Source: CAD feature listing. Evaluate the final solid. Frame: model axes, mm. A direction names the side the tool comes from. Coordinates: 2 decimals unless noted, no trailing zeros. Write each loop counter-clockwise with the first axis right and the second up, starting at its lowest first coordinate (ties: lowest second). Pieces come first, ordered by that corner, then holes. Notation, with made-up numbers: (76, -19) - (118, -19) arc R30 cw to (118, 13) - close; hole circle Ø1 at (0.25, 78). An arc over 180 degrees is marked (long way). One line per item, written item: value.
from build123d import *

# Parameters (mm, degrees)
F1_DEPTH  = 5.5372
F3_D      = 57.8866
F5_DEPTH  = 5.5382
F7_DEPTH  = 17.76331
F9_DEPTH  = 25.4
F11_DEPTH = 25.4
F13_DEPTH = 25.4


with BuildPart() as f1:
    # F0 (on Front) → F1 (new body)
    with BuildSketch(Plane.XZ):
        Polygon((85.176131, 104.177512), (-67.223869, 104.177512), (-143.423869, -1.364378), (-143.423869, -52.164378), (161.376131, -52.164378), (161.376131, -1.364378), align=None)
    extrude(amount=F1_DEPTH)

    # F3 (through all)
    with Locations(Plane.XZ.offset(5.5372)):
        with Locations((-41.244327, 53.377512), (59.196589, 53.377512), (110.576131, 2.577512), (8.976131, 2.577512), (-92.623869, 2.577512)):
            Hole(F3_D / 2)

    # F4 (on face) → F5 (cut, through all)
    with BuildSketch(Plane.XZ.offset(5.5372)):
        with BuildLine():
            ThreePointArc((-87.315269, -35.095578), (-88.140769, -34.270078), (-88.966269, -35.095578))
            Line((-88.966269, -35.095578), (-88.966269, -43.985578))
            Line((-88.966269, -43.985578), (-71.516469, -43.985578))
            Line((-71.516469, -43.985578), (-71.516469, -35.095578))
            ThreePointArc((-71.516469, -35.095578), (-72.341969, -34.270078), (-73.167469, -35.095578))
            Line((-73.167469, -35.095578), (-73.167469, -41.597978))
            Line((-73.167469, -41.597978), (-87.315269, -41.597978))
            Line((-87.315269, -41.597978), (-87.315269, -35.095578))
        make_face()
    extrude(amount=-F5_DEPTH, mode=Mode.SUBTRACT)

    # F6 (on face) → F7 (cut)
    with BuildSketch(Plane.XZ.offset(5.5372)):
        with BuildLine():
            ThreePointArc((-43.424069, -35.095578), (-44.249569, -34.270078), (-45.075069, -35.095578))
            Line((-45.075069, -35.095578), (-45.075069, -43.985578))
            Line((-45.075069, -43.985578), (-27.625269, -43.985578))
            Line((-27.625269, -43.985578), (-27.625269, -35.095578))
            ThreePointArc((-27.625269, -35.095578), (-28.450769, -34.270078), (-29.276269, -35.095578))
            Line((-29.276269, -35.095578), (-29.276269, -41.597978))
            Line((-29.276269, -41.597978), (-43.424069, -41.597978))
            Line((-43.424069, -41.597978), (-43.424069, -35.095578))
        make_face()
    extrude(amount=-F7_DEPTH, mode=Mode.SUBTRACT)

    # F8 (on face) → F9 (cut)
    with BuildSketch(Plane.XZ.offset(5.5372)):
        with BuildLine():
            ThreePointArc((1.076731, -35.095578), (0.251231, -34.270078), (-0.574269, -35.095578))
            Line((-0.574269, -35.095578), (-0.574269, -43.985578))
            Line((-0.574269, -43.985578), (16.875531, -43.985578))
            Line((16.875531, -43.985578), (16.875531, -35.095578))
            ThreePointArc((16.875531, -35.095578), (16.050031, -34.270078), (15.224531, -35.095578))
            Line((15.224531, -35.095578), (15.224531, -41.597978))
            Line((15.224531, -41.597978), (1.076731, -41.597978))
            Line((1.076731, -41.597978), (1.076731, -35.095578))
        make_face()
    extrude(amount=-F9_DEPTH, mode=Mode.SUBTRACT)

    # F10 (on face) → F11 (cut)
    with BuildSketch(Plane.XZ.offset(5.5372)):
        with BuildLine():
            ThreePointArc((47.228531, -35.095578), (46.403031, -34.270078), (45.577531, -35.095578))
            Line((45.577531, -35.095578), (45.577531, -43.985578))
            Line((45.577531, -43.985578), (63.027331, -43.985578))
            Line((63.027331, -43.985578), (63.027331, -35.095578))
            ThreePointArc((63.027331, -35.095578), (62.201831, -34.270078), (61.376331, -35.095578))
            Line((61.376331, -35.095578), (61.376331, -41.597978))
            Line((61.376331, -41.597978), (47.228531, -41.597978))
            Line((47.228531, -41.597978), (47.228531, -35.095578))
        make_face()
    extrude(amount=-F11_DEPTH, mode=Mode.SUBTRACT)

    # F12 (on face) → F13 (cut)
    with BuildSketch(Plane.XZ.offset(5.5372)):
        with BuildLine():
            ThreePointArc((91.119731, -35.095578), (90.294231, -34.270078), (89.468731, -35.095578))
            Line((89.468731, -35.095578), (89.468731, -43.985578))
            Line((89.468731, -43.985578), (106.918531, -43.985578))
            Line((106.918531, -43.985578), (106.918531, -35.095578))
            ThreePointArc((106.918531, -35.095578), (106.093031, -34.270078), (105.267531, -35.095578))
            Line((105.267531, -35.095578), (105.267531, -41.597978))
            Line((105.267531, -41.597978), (91.119731, -41.597978))
            Line((91.119731, -41.597978), (91.119731, -35.095578))
        make_face()
    extrude(amount=-F13_DEPTH, mode=Mode.SUBTRACT)


solid = f1.part
1) Section query B-B on x = 133. Output: boundary loops of the cut face in (y, z).
Values found:
outline: (-5.54, -52.16) - (0, -52.16) - (0, -15.72) - (-5.54, -15.72) - close; (-5.54, 20.88) - (0, 20.88) - (0, 37.94) - (-5.54, 37.94) - close
2) Section query D-D on z = 12. Output: boundary loops of the cut face in (x, y).
Values found:
outline: (-133.77, -5.54) - (-119.99, -5.54) - (-119.99, 0) - (-133.77, 0) - close; (-65.26, -5.54) - (-18.39, -5.54) - (-18.39, 0) - (-65.26, 0) - close; (36.34, -5.54) - (83.21, -5.54) - (83.21, 0) - (36.34, 0) - close; (137.94, -5.54) - (151.73, -5.54) - (151.73, 0) - (137.94, 0) - close
3) Section query A-A on z = 43.5. Output: boundary loops of the cut face in (x, y), then the cut area to 3 significant figures.
Values found:
outline: (-111.03, -5.54) - (-68.45, -5.54) - (-68.45, 0) - (-111.03, 0) - close; (-14.04, -5.54) - (31.99, -5.54) - (31.99, 0) - (-14.04, 0) - close; (86.4, -5.54) - (128.98, -5.54) - (128.98, 0) - (86.4, 0) - close
area: 726 mm2
4) Draft query along Z for faces 3 (the flat face through (123.81, -2.73, 50.67)), 4 (the flat face through (-36, -3, -41.598)), 5 (the flat face through (7, 0, 44)). Return one class per face: released by +Z, released by -Z, zero draft, split by the parting line, or undercut.
Values found:
face 3: released by +Z
face 4: undercut
face 5: zero draft
5) Reachability of faces 1 (the flat face through (89.469, -3, -39)), 2 (the flat face through (-143.424, -3, -26)) from +Z, -Z, +X, -X, +Y, -Y: full face, straight path, thin tool, end or side. Return the list, or none.
Values found:
face 1: +Y, -Y
face 2: +Z, -Z, -X, +Y, -Y
6) Material intervals for line 1 (X direction, y = -1.2, z = 10.5); line 2 (X direction, y = -4.7, z = 71); line 3 (X direction, y = -3, z = -13.5), sorted ascending.
Values found:
line 1: -134.86 to -120.46, -64.79 to -18.86, 36.81 to 82.74, 138.41 to 152.81
line 2: -91.18 to -64.2, -18.28 to 36.24, 82.16 to 109.13
line 3: -143.42 to -116.69, -68.56 to -15.09, 33.04 to 86.51, 134.64 to 161.38
7) Contact query for flat-ended pins moving along their axis: P1, Ø1.7, axis at x = 96, y = -3.5, coming from the +Z side; P2, Ø2, axis at y = -3.5, z = 0, coming from the +X side; P3, Ø1.5, axis at x = -90, y = -1, coming from the +Z side. Output: stop coordinate, or through.
Values found:
P1: z = 90.36
P2: x = 161.11
P3: z = 73.67
8) Section query C-C on x = -77. Output: boundary loops of the cut face in (y, z), then the cut area to 3 significant figures.
Values found:
outline: (-5.54, -52.16) - (0, -52.16) - (0, -43.99) - (-5.54, -43.99) - close; (-5.54, -41.6) - (0, -41.6) - (0, -21.79) - (-5.54, -21.79) - close; (-5.54, 26.94) - (0, 26.94) - (0, 90.64) - (-5.54, 90.64) - close
area: 508 mm2
